Autodesk Inventor part; units mm, degrees
ref_plane "YZ Plane" through (0, 0, 0) normal (1, 0, 0) x (0, 1, 0)
ref_plane "XZ Plane" through (0, 0, 0) normal (0, 1, 0) x (-1, 0, 0)
ref_plane "XY Plane" through (0, 0, 0) normal (0, 0, 1) x (1, 0, 0)
sketch "Sketch1" plane through (0, 0, 0) normal (0, 0, 1) x (1, 0, 0)
  line L0 (-2.0207, 3.5005) -> (2.0207, 3.5005)
  line L1 (2.0207, 3.5005) -> (4.0415, 0.0005)
  line L2 (-4.0415, 0.0005) -> (-2.0207, 3.5005)
  line L3 (-2.0207, -3.4995) -> (-4.0415, 0.0005)
  line L4 (4.0415, 0.0005) -> (2.0207, -3.4995)
  line L5 (2.0207, -3.4995) -> (-2.0207, -3.4995)
  line L6 (-11.749, 11.7485) -> (11.751, 11.7485)
  line L7 (11.751, 11.7485) -> (11.751, -11.7515)
  line L8 (11.751, -11.7515) -> (-11.749, -11.7515)
  line L9 (-11.749, -11.7515) -> (-11.749, 11.7485)
  point P0 (0, 0)
  point P1 (0.001, -0.0015)
  dimension "d7" = 23.5
  dimension "d8" = 23.5
extrude "Extrusion1" add sketch "Sketch1" along normal blind 3
properties part number "hex slot holder" material "Gold"
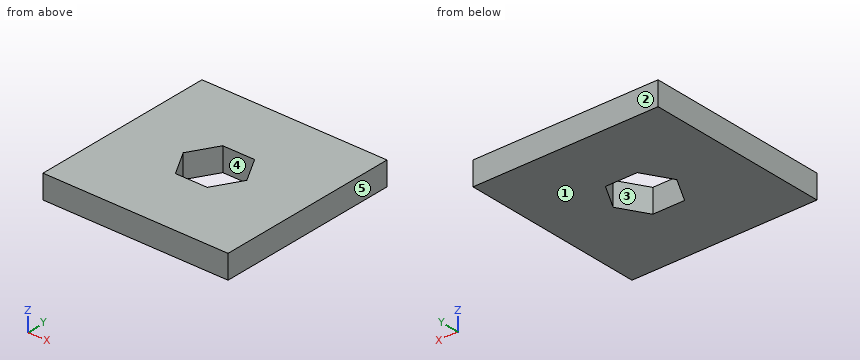
Check sheet for the modelled part. Datum: model origin and axes. Units: mm. Face numbers are marked on the shaded views. A direction names the side the tool comes from. Round coordinates to 2 decimals unless told otherwise and drop trailing zeros. Loops run counter-clockwise (first coordinate to the right, second up) from the corner with the lowest first, then second, coordinate; pieces in that order, holes last. Notation, with made-up numbers: (18.5, 47) - (30.5, 47) arc R25 cw to (30.5, 62) - close; hole circle Ø3 at (51, 56). An arc over 180 degrees is marked (long way). Write item = value, one per line. Start each with the question number.
Q1. Release check for a two-part mould opening along Y. For the marked faces 1, 2 and 3 record: pulls with the +Y half, pulls with the -Y half, needs draft (parallel to the pull), parting line crosses it, or undercut.
Q2. Depth check by flat-ended pin: P1, Ø8, axis at x = 6.5, y = 6, coming from the -Z side. Enter the tip coordinate at first touch or a pass-through.
Q3. Section check A-A (x = 1.5). Record the boundary of the cut face in (y, z).
Q4. Section check B-B (z = 0.6). Record the boundary of the cut face in (x, y).
Q5. Thickness scan on L1, parallel to Y at x = 0.25, z = 2.4; L2, parallel to X at y = -2.5, z = 1.5; L3, parallel to Y at x = -3.5, z = 0.45. Record the ranges inside material, lowest first.
Q6. Access from +Z, -Z, +X, -X, +Y, -Y to the whole of each face (thin tool, end or side, straight path). Record for the marked faces 4 and 5.
Q7. Section check C-C (y = 1). Record the boundary of the cut face in (x, z).
Derived:
q1.face_1 = needs draft
q1.face_2 = pulls with the +Y half
q1.face_3 = undercut
q2.P1 = 0
q3.outline = (-11.75, 0) - (-3.5, 0) - (-3.5, 3) - (-11.75, 3) - close; (3.5, 0) - (11.75, 0) - (11.75, 3) - (3.5, 3) - close
q4.outline = (-11.75, -11.75) - (11.75, -11.75) - (11.75, 11.75) - (-11.75, 11.75) - close; hole (-4.04, 0) - (-2.02, -3.5) - (2.02, -3.5) - (4.04, 0) - (2.02, 3.5) - (-2.02, 3.5) - close
q5.L1 = -11.75 to -3.5, 3.5 to 11.75
q5.L2 = -11.75 to -2.6, 2.6 to 11.75
q5.L3 = -11.75 to -0.94, 0.94 to 11.75
q6.face_4 = +Z, -Z
q6.face_5 = +Z, -Z, +X, +Y, -Y
q7.outline = (-11.75, 0) - (-3.46, 0) - (-3.46, 3) - (-11.75, 3) - close; (3.46, 0) - (11.75, 0) - (11.75, 3) - (3.46, 3) - close
